from build123d import *

# Parameters (mm, degrees)
F0_R          = 21
F1_DEPTH      = 5
F2_R          = 18.5
F3_DEPTH      = 6.2
F5_DEPTH      = 6.2
F5_DEPTH_BACK = 5
F6_SIZE       = 0.1


with BuildPart() as f1:
    # F0 (on Front) → F1 (new body)
    with BuildSketch(Plane.XZ):
        Circle(F0_R)
    extrude(amount=-F1_DEPTH)

    # F2 (on Front) → F3 (join)
    with BuildSketch(Plane.XZ):
        Circle(F2_R)
    extrude(amount=F3_DEPTH)

    # F4 (on Front) → F5 (cut, two sides)
    with BuildSketch(Plane.XZ) as f5_sk:
        with BuildLine():
            ThreePointArc((7.7074639149, 7.7074639149), (9.4511282566, 7.3606275128), (10.4388347648, 8.8388347648))
            ThreePointArc((10.4388347648, 8.8388347648), (10.3170420168, 9.4511282566), (9.9702056147, 9.9702056147))
            Line((9.9702056147, 9.9702056147), (7.7074639149, 7.7074639149))
        make_face()
        with BuildLine():
            ThreePointArc((12.3530483272, -10.2530483272), (11.0566835352, -8.3129013089), (8.7681240867, -8.7681240867))
            Line((8.7681240867, -8.7681240867), (11.7379725677, -11.7379725677))
            ThreePointArc((11.7379725677, -11.7379725677), (12.1931953455, -11.0566835352), (12.3530483272, -10.2530483272))
        make_face()
        with BuildLine():
            Line((11.7379725677, -11.7379725677), (8.7681240867, -8.7681240867))
            ThreePointArc((8.7681240867, -8.7681240867), (8.7681240867, -11.7379725677), (11.7379725677, -11.7379725677))
        make_face()
        with BuildLine():
            ThreePointArc((-7.2388347648, -8.8388347648), (-7.3606275128, -8.226541273), (-7.7074639149, -7.7074639149))
            Line((-7.7074639149, -7.7074639149), (-9.9702056147, -9.9702056147))
            ThreePointArc((-9.9702056147, -9.9702056147), (-8.226541273, -10.3170420168), (-7.2388347648, -8.8388347648))
        make_face()
        with BuildLine():
            Line((-9.9702056147, -9.9702056147), (-7.7074639149, -7.7074639149))
            ThreePointArc((-7.7074639149, -7.7074639149), (-9.9702056147, -7.7074639149), (-9.9702056147, -9.9702056147))
        make_face()
        with BuildLine():
            ThreePointArc((-11.7379725677, 11.7379725677), (-11.7379725677, 8.7681240867), (-8.7681240867, 8.7681240867))
            Line((-8.7681240867, 8.7681240867), (-11.7379725677, 11.7379725677))
        make_face()
        with BuildLine():
            Line((-11.7379725677, 11.7379725677), (-8.7681240867, 8.7681240867))
            ThreePointArc((-8.7681240867, 8.7681240867), (-8.3129013089, 9.4494131192), (-8.1530483272, 10.2530483272))
            ThreePointArc((-8.1530483272, 10.2530483272), (-9.4494131192, 12.1931953455), (-11.7379725677, 11.7379725677))
        make_face()
        with BuildLine():
            ThreePointArc((8.75, 0), (8.0839459095, 3.3484800332), (6.1871843354, 6.1871843354))
            Line((6.1871843354, 6.1871843354), (0, 0))
            Line((0, 0), (6.1871843354, -6.1871843354))
            ThreePointArc((6.1871843354, -6.1871843354), (8.0839459095, -3.3484800332), (8.75, 0))
        make_face()
        with BuildLine():
            Line((0, 0), (6.1871843354, 6.1871843354))
            ThreePointArc((6.1871843354, 6.1871843354), (0, 8.75), (-6.1871843354, 6.1871843354))
            Line((-6.1871843354, 6.1871843354), (0, 0))
        make_face()
        with BuildLine():
            Line((7.7074639149, 7.7074639149), (9.9702056147, 9.9702056147))
            ThreePointArc((9.9702056147, 9.9702056147), (7.7074639149, 9.9702056147), (7.7074639149, 7.7074639149))
        make_face()
        with BuildLine():
            Line((0, 0), (-6.1871843354, 6.1871843354))
            ThreePointArc((-6.1871843354, 6.1871843354), (-8.75, 0), (-6.1871843354, -6.1871843354))
            Line((-6.1871843354, -6.1871843354), (0, 0))
        make_face()
        with BuildLine():
            Line((6.1871843354, -6.1871843354), (0, 0))
            Line((0, 0), (-6.1871843354, -6.1871843354))
            ThreePointArc((-6.1871843354, -6.1871843354), (0, -8.75), (6.1871843354, -6.1871843354))
        make_face()
    extrude(amount=F5_DEPTH, mode=Mode.SUBTRACT)
    extrude(f5_sk.sketch, amount=-F5_DEPTH_BACK, mode=Mode.SUBTRACT)

    # F6
    f6_edges = [f1.edges().sort_by_distance(p)[0] for p in [
        (-21, 5, 0),
        (-9.970206, 5, -9.970206),
        (11.737973, 5, -11.737973),
        (6.187184, 5, 6.187184),
        (-11.737973, 5, 11.737973),
        (7.707464, 5, 7.707464),
        (-21, 0, 0),
    ]]
    chamfer(f6_edges, length=F6_SIZE)


solid = f1.part
Could you check a few things on this model? Use its own coordinates, in mm. A direction names the side the tool comes from. Give positions to 0.01 mm unless a question says otherwise; leave off trailing zeros. Order: outer loops, then holes, each group sorted by start corner. A loop starts at its lowest first (then second) coordinate and runs counter-clockwise, first axis right, second up. Notation, with made-up numbers: (13, -28) -> (18, -28) arc R8 cw to (18, -21) -> close; hole circle Ø7 at (41, 85.25). An arc over 180 degrees is marked (long way). Answer in a Markdown table with one row per item. Add a question column.
Item 1: Imagine slicing it at B-B (y = -3). List the corners of the cut face in (x, z) for me, and give its area (3 significant figures).
Item 2: Imagine slicing it at A-A (x = 0). List the corners of the cut face in (y, z) for me, and give its area (3 significant figures).
Item 3: I'm going to push flat-ended pins straight in: P1, Ø2, axis at x = 2, y = -4, coming from the +Z side; P2, Ø5, axis at y = -4, z = -3.5, coming from the +X side; P3, Ø4, axis at y = -3.5, z = -13.5, coming from the -X side. Where does each tip first touch, or does it pass through?
Item 4: Imagine slicing it at C-C (y = 2.5). List the corners of the cut face in (x, z) for me, and give its area (3 significant figures).
Item 5: For faces 1 (the cylindrical face through (20.03, 2.47, 6.31)), 2 (the cylindrical face through (-4.01, -3.06, -18.06)), which set-ups out of +Z, -Z, +X, -X, +Y, -Y let a thin tool reach every point of the face, with its end or its side?
Item 6: Please list where these lines run through material, in increasing order: probe 1 along Z at (x, y) = (10, -3); probe 2 along X at (y, z) = (1.5, -10); probe 3 along Z at (x, y) = (-7, -0.5).
Result:
| question | item | result |
|---|---|---|
| 1 | outline | circle Ø37 at (0, 0); hole circle Ø4.2 at (-10.25, 10.25); hole circle Ø3.2 at (-8.84, -8.84); hole circle Ø17.5 at (0, 0); hole circle Ø3.2 at (8.84, 8.84); hole circle Ø4.2 at (10.25, -10.25) |
| 1 | area | 791 mm2 |
| 2 | outline | (-6.2, -18.5) -> (0, -18.5) -> (0, -20.9) -> (0.1, -21) -> (4.9, -21) -> (5, -20.9) -> (5, -8.85) -> (4.9, -8.75) -> (-6.2, -8.75) -> close; (-6.2, 8.75) -> (4.9, 8.75) -> (5, 8.85) -> (5, 20.9) -> (4.9, 21) -> (0.1, 21) -> (0, 20.9) -> (0, 18.5) -> (-6.2, 18.5) -> close |
| 2 | area | 243 mm2 |
| 3 | P1 | z = 18.47 |
| 3 | P2 | x = 18.47 |
| 3 | P3 | x = -14.49 |
| 4 | outline | circle Ø42 at (0, 0); hole circle Ø4.2 at (-10.25, 10.25); hole circle Ø3.2 at (-8.84, -8.84); hole circle Ø17.5 at (0, 0); hole circle Ø3.2 at (8.84, 8.84); hole circle Ø4.2 at (10.25, -10.25) |
| 4 | area | 1,100 mm2 |
| 5 | face 1 | +Y, -Y |
| 5 | face 2 | -Y |
| 6 | probe 1 | -15.56 to -12.34, -8.17 to 7.74, 9.94 to 15.56 |
| 6 | probe 2 | -18.47 to -9.94, -7.74 to 8.17, 12.34 to 18.47 |
| 6 | probe 3 | -17.12 to -5.25, 5.25 to 17.12 |
